```python
from build123d import *

# Parameters (mm, degrees)
SKETCH1_W                    = 320
SKETCH1_H                    = 90.51
CHASSIS_BASE_DEPTH           = 5
SKETCH3_W                    = 2
SKETCH3_H                    = 275
LATERAL_GUARD_DEPTH          = 3
DRIVE_ATTACHMENT_POINT_REACH = 168.469
SKETCH4_R                    = 3
CUT_EXTRUDE2_REACH           = 168.352
SKETCH5_R                    = 6.5
SKETCH5_R_2                  = 1
SKETCH6_W                    = 20
SKETCH6_H                    = 20
BOSS_EXTRUDE1_DEPTH          = 90.51
CUT_EXTRUDE3_REACH           = 169.475
SKETCH7_W                    = 60
SKETCH7_H                    = 23.073600821
FILLET3_R                    = 0.5
FILLET4_R                    = 2
SKETCH9_R                    = 0.875
CUT_EXTRUDE5_DEPTH           = 5
SKETCH10_R                   = 0.875
CUT_EXTRUDE6_DEPTH           = 5
SKETCH11_R                   = 0.875
CUT_EXTRUDE7_DEPTH           = 5
SKETCH12_R                   = 0.875
CUT_EXTRUDE8_DEPTH           = 5
SKETCH13_R                   = 0.875
CUT_EXTRUDE9_DEPTH           = 5
SKETCH14_R                   = 0.875
CUT_EXTRUDE10_DEPTH          = 5
BOSS_EXTRUDE2_DEPTH          = 1.6


with BuildPart() as part:
    # Sketch1 → Chassis Base (new body)
    with BuildSketch(Plane(origin=(0, 0, 0), x_dir=(0, 1, 0), z_dir=(0, 0, 1))):
        Rectangle(SKETCH1_W, SKETCH1_H)
    extrude(amount=CHASSIS_BASE_DEPTH)

    # Sketch3 → Lateral Guard (add)
    with BuildSketch(Plane.XY.offset(5)):
        with Locations((-44.255, 7.5)):
            Rectangle(SKETCH3_W, SKETCH3_H)
        with Locations((44.255, 7.5)):
            Rectangle(SKETCH3_W, SKETCH3_H)
    extrude(amount=LATERAL_GUARD_DEPTH)

    # Sketch4 → Drive Attachment Point (cut, up to next)
    with BuildSketch(Plane(origin=(0, 0, 0), x_dir=(1, 0, 0), z_dir=(0, 0, -1)), mode=Mode.PRIVATE) as drive_attachment_point_sk1:
        with Locations(Location((0, -29.7, 0), (0, 0, 180))):
            Circle(SKETCH4_R)
    drive_attachment_point_tool1 = extrude(drive_attachment_point_sk1.sketch, amount=-DRIVE_ATTACHMENT_POINT_REACH, mode=Mode.PRIVATE) & part.part
    # Sketch4 → Drive Attachment Point (cut, up to next)
    with BuildSketch(Plane(origin=(0, 0, 0), x_dir=(1, 0, 0), z_dir=(0, 0, -1)), mode=Mode.PRIVATE) as drive_attachment_point_sk2:
        with Locations(Location((-20.08, 30, 0), (0, 0, 180))):
            Circle(SKETCH4_R)
    drive_attachment_point_tool2 = extrude(drive_attachment_point_sk2.sketch, amount=-DRIVE_ATTACHMENT_POINT_REACH, mode=Mode.PRIVATE) & part.part
    # Sketch4 → Drive Attachment Point (cut, up to next)
    with BuildSketch(Plane(origin=(0, 0, 0), x_dir=(1, 0, 0), z_dir=(0, 0, -1)), mode=Mode.PRIVATE) as drive_attachment_point_sk3:
        with Locations((20.08, 30)):
            Circle(SKETCH4_R)
    drive_attachment_point_tool3 = extrude(drive_attachment_point_sk3.sketch, amount=-DRIVE_ATTACHMENT_POINT_REACH, mode=Mode.PRIVATE) & part.part
    # Sketch4 → Drive Attachment Point (cut, up to next)
    with BuildSketch(Plane(origin=(0, 0, 0), x_dir=(1, 0, 0), z_dir=(0, 0, -1)), mode=Mode.PRIVATE) as drive_attachment_point_sk4:
        with Locations(Location((0, 49.3, 0), (0, 0, 180))):
            Circle(SKETCH4_R)
    drive_attachment_point_tool4 = extrude(drive_attachment_point_sk4.sketch, amount=-DRIVE_ATTACHMENT_POINT_REACH, mode=Mode.PRIVATE) & part.part
    # Sketch4 → Drive Attachment Point (cut, up to next)
    with BuildSketch(Plane(origin=(0, 0, 0), x_dir=(1, 0, 0), z_dir=(0, 0, -1)), mode=Mode.PRIVATE) as drive_attachment_point_sk5:
        with Locations(Location((-20.08, -10.4, 0), (0, 0, 180))):
            Circle(SKETCH4_R)
    drive_attachment_point_tool5 = extrude(drive_attachment_point_sk5.sketch, amount=-DRIVE_ATTACHMENT_POINT_REACH, mode=Mode.PRIVATE) & part.part
    # Sketch4 → Drive Attachment Point (cut, up to next)
    with BuildSketch(Plane(origin=(0, 0, 0), x_dir=(1, 0, 0), z_dir=(0, 0, -1)), mode=Mode.PRIVATE) as drive_attachment_point_sk6:
        with Locations(Location((20.08, -10.4, 0), (0, 0, 180))):
            Circle(SKETCH4_R)
    drive_attachment_point_tool6 = extrude(drive_attachment_point_sk6.sketch, amount=-DRIVE_ATTACHMENT_POINT_REACH, mode=Mode.PRIVATE) & part.part
    add(drive_attachment_point_tool1.solids().sort_by_distance((0, 29.7, 0))[0], mode=Mode.SUBTRACT)
    add(drive_attachment_point_tool2.solids().sort_by_distance((-20.08, -30, 0))[0], mode=Mode.SUBTRACT)
    add(drive_attachment_point_tool3.solids().sort_by_distance((20.08, -30, 0))[0], mode=Mode.SUBTRACT)
    add(drive_attachment_point_tool4.solids().sort_by_distance((0, -49.3, 0))[0], mode=Mode.SUBTRACT)
    add(drive_attachment_point_tool5.solids().sort_by_distance((-20.08, 10.4, 0))[0], mode=Mode.SUBTRACT)
    add(drive_attachment_point_tool6.solids().sort_by_distance((20.08, 10.4, 0))[0], mode=Mode.SUBTRACT)

    # Sketch5 → Cut-Extrude2 (cut, up to next)
    with BuildSketch(Plane.XY.offset(5), mode=Mode.PRIVATE) as cut_extrude2_sk1:
        with Locations((0, 148)):
            Circle(SKETCH5_R)
    cut_extrude2_tool1 = extrude(cut_extrude2_sk1.sketch, amount=-CUT_EXTRUDE2_REACH, mode=Mode.PRIVATE) & part.part
    # Sketch5 → Cut-Extrude2 (cut, up to next)
    with BuildSketch(Plane.XY.offset(5), mode=Mode.PRIVATE) as cut_extrude2_sk2:
        with Locations((-17.5, 140.5)):
            Circle(SKETCH5_R_2)
    cut_extrude2_tool2 = extrude(cut_extrude2_sk2.sketch, amount=-CUT_EXTRUDE2_REACH, mode=Mode.PRIVATE) & part.part
    # Sketch5 → Cut-Extrude2 (cut, up to next)
    with BuildSketch(Plane.XY.offset(5), mode=Mode.PRIVATE) as cut_extrude2_sk3:
        with Locations((17.5, 140.5)):
            Circle(SKETCH5_R_2)
    cut_extrude2_tool3 = extrude(cut_extrude2_sk3.sketch, amount=-CUT_EXTRUDE2_REACH, mode=Mode.PRIVATE) & part.part
    add(cut_extrude2_tool1.solids().sort_by_distance((0, 148, 5))[0], mode=Mode.SUBTRACT)
    add(cut_extrude2_tool2.solids().sort_by_distance((-17.5, 140.5, 5))[0], mode=Mode.SUBTRACT)
    add(cut_extrude2_tool3.solids().sort_by_distance((17.5, 140.5, 5))[0], mode=Mode.SUBTRACT)

    # Sketch6 → Boss-Extrude1 (add)
    with BuildSketch(Plane.YZ.offset(45.255)):
        with Locations((-150, 10)):
            Rectangle(SKETCH6_W, SKETCH6_H)
    extrude(amount=-BOSS_EXTRUDE1_DEPTH)

    # Sketch7 → Cut-Extrude3 (cut, up to next)
    with BuildSketch(Plane.XY.offset(20), mode=Mode.PRIVATE) as cut_extrude3_sk1:
        with Locations((0, -148.463199589)):
            Rectangle(SKETCH7_W, SKETCH7_H)
    cut_extrude3_tool1 = extrude(cut_extrude3_sk1.sketch, amount=-CUT_EXTRUDE3_REACH, mode=Mode.PRIVATE) & part.part
    add(cut_extrude3_tool1.solids().sort_by_distance((0, -148.4632, 20))[0], mode=Mode.SUBTRACT)

    # Fillet3
    fillet3_edges = [part.edges().sort_by_distance(p)[0] for p in [
        (-45.255, 7.5, 8),
        (-43.255, 7.5, 8),
        (45.255, 7.5, 8),
        (43.255, 7.5, 8),
    ]]
    fillet(fillet3_edges, radius=FILLET3_R)

    # Fillet4
    fillet4_edges = [part.edges().sort_by_distance(p)[0] for p in [
        (37.6275, -140, 20),
        (-37.6275, -140, 20),
    ]]
    fillet(fillet4_edges, radius=FILLET4_R)

    # Sketch9 → Cut-Extrude5 (cut)
    with BuildSketch(Plane.XY.offset(20)):
        with Locations((-37.6275, -151)):
            Circle(SKETCH9_R)
    extrude(amount=-CUT_EXTRUDE5_DEPTH, mode=Mode.SUBTRACT)

    # Sketch10 → Cut-Extrude6 (cut)
    with BuildSketch(Plane.XZ.offset(160)):
        with Locations(Location((-37.6275, 10, 0), (0, 0, 270))):
            Circle(SKETCH10_R)
    extrude(amount=-CUT_EXTRUDE6_DEPTH, mode=Mode.SUBTRACT)

    # Sketch11 → Cut-Extrude7 (cut)
    with BuildSketch(Plane(origin=(0, 0, 0), x_dir=(1, 0, 0), z_dir=(0, 0, -1))):
        with Locations(Location((-37.6275, 148.599605515, 0), (0, 0, 180))):
            Circle(SKETCH11_R)
    extrude(amount=-CUT_EXTRUDE7_DEPTH, mode=Mode.SUBTRACT)

    # Sketch12 → Cut-Extrude8 (cut)
    with BuildSketch(Plane(origin=(0, 0, 0), x_dir=(1, 0, 0), z_dir=(0, 0, -1))):
        with Locations(Location((37.6275, 148.463199589, 0), (0, 0, 180))):
            Circle(SKETCH12_R)
    extrude(amount=-CUT_EXTRUDE8_DEPTH, mode=Mode.SUBTRACT)

    # Sketch13 → Cut-Extrude9 (cut)
    with BuildSketch(Plane.XZ.offset(160)):
        with Locations(Location((37.6275, 10, 0), (0, 0, 270))):
            Circle(SKETCH13_R)
    extrude(amount=-CUT_EXTRUDE9_DEPTH, mode=Mode.SUBTRACT)

    # Sketch14 → Cut-Extrude10 (cut)
    with BuildSketch(Plane.XY.offset(20)):
        with Locations((37.6275, -151)):
            Circle(SKETCH14_R)
    extrude(amount=-CUT_EXTRUDE10_DEPTH, mode=Mode.SUBTRACT)

    # Sketch15 → Boss-Extrude2 (add)
    with BuildSketch(Plane.XY.offset(5)):
        with BuildLine():
            Line((-17.021586315, 136.436061109), (17.021586315, 136.436061109))
            ThreePointArc((17.021586315, 136.436061109), (0, 123), (-17.021586315, 136.436061109))
        make_face()
    extrude(amount=BOSS_EXTRUDE2_DEPTH)


solid = part.part
```
Check sheet for the modelled part. Datum: model origin and axes. Units: mm. A direction names the side the tool comes from. Coordinates: 2 decimals unless noted, no trailing zeros. Order: outer loops, then holes, each group sorted by start corner. A loop starts at its lowest first (then second) coordinate and runs counter-clockwise, first axis right, second up. Notation, with made-up numbers: M -36.5,44 L 6.5,44 A16 ccw 6.5,70 Z; hole C 49.25,4.5 d10. An arc over 180 degrees is marked long. One line per question, with ' | ' between items. Start each with the question number.
Item 1: Sectioned sample at A-A on y = 148. Record the cut outline in (x, z) (3 decimals), and give its area (3 significant figures).
Item 2: Sectioned sample at C-C on x = 13. Record the cut outline in (y, z), and give its area (3 significant figures).
Item 3: Mould release check, pull along Y, two halves, no side actions. Record for faces 1 (the cylindrical face through (0.391, 32.674, 2.465)), 2 (the flat face through (-39, -160, 10)), 3 (the flat face through (-36, -151, 20)): pulls with the +Y half, pulls with the -Y half, needs draft (parallel to the pull), parting line crosses it, or undercut.
Item 4: Material ranges on line 1 (Y direction, x = -20.08, z = 2); line 2 (X direction, y = -151, z = 17.7) (1 decimal); line 3 (X direction, y = 140.5, z = 3.45) (3 decimals), recorded low to high.
Item 5: Sectioned sample at D-D on y = -22.5. Record the cut outline in (x, z) (3 decimals), and give its area (3 significant figures).
Item 6: Sectioned sample at B-B on y = 10.4. Record the cut outline in (x, z) (3 decimals).
Item 7: Access from +Z, -Z, +X, -X, +Y, -Y to the whole of each face (thin tool, end or side, straight path). Record for faces 4 (the flat face through (0, 131, 6.6)), 5 (the flat face through (-30, -149, 10)), 6 (the cylindrical face through (0, 123, 6)), 7 (the cylindrical face through (0.391, -46.326, 2.465)).
Item 8: Gauge pin test, flat ends, axial feed: P1, Ø4, axis at x = 0.5, z = 1.5, coming from the -Y side; P2, Ø6.5, axis at x = 36.5, z = 13.5, coming from the +Y side; P3, Ø0.8, axis at x = 0.5, z = 6, coming from the +Y side. Record the tip position at first contact, or that the pin passes through.
Answer below:
1) outline: M -45.255,0 L -6.5,0 L -6.5,5 L -45.255,5 Z; M 6.5,0 L 45.255,0 L 45.255,5 L 6.5,5 Z | area: 388 mm^2
2) outline: M -136.93,0 L 160,0 L 160,5 L 136.44,5 L 136.44,6.6 L 128.78,6.6 L 128.78,5 L -136.93,5 Z | area: 1,500 mm^2
3) face 1: undercut | face 2: pulls with the -Y half | face 3: needs draft
4) line 1: y = -136.93 to -33, -27 to 7.4, 13.4 to 160 | line 2: x = -45.3 to -38.5, -36.8 to -30, 30 to 36.8, 38.5 to 45.3 | line 3: x = -45.255 to -18.5, -16.5 to 16.5, 18.5 to 45.255
5) outline: M -45.255,0 L 45.255,0 L 45.255,7.5 A0.5 ccw 44.755,8 L 43.755,8 A0.5 ccw 43.255,7.5 L 43.255,5 L -43.255,5 L -43.255,7.5 A0.5 ccw -43.755,8 L -44.755,8 A0.5 ccw -45.255,7.5 Z | area: 464 mm^2
6) outline: M -45.255,0 L -23.08,0 L -23.08,5 L -43.255,5 L -43.255,7.5 A0.5 ccw -43.755,8 L -44.755,8 A0.5 ccw -45.255,7.5 Z; M -17.08,0 L 17.08,0 L 17.08,5 L -17.08,5 Z; M 23.08,0 L 45.255,0 L 45.255,7.5 A0.5 ccw 44.755,8 L 43.755,8 A0.5 ccw 43.255,7.5 L 43.255,5 L 23.08,5 Z
7) face 4: +Z, +Y, -Y | face 5: +Z, -Z, -Y | face 6: +Z, -Y | face 7: +Z, -Z
8) P1: stops at y = -136.93 | P2: stops at y = -140 | P3: stops at y = 136.44
